Geometry check sheet. Reference: drawing and pictorial views, mm from the part's lowest x, y, z. A direction names the side the tool comes from. Give positions to 0.01 mm unless a question says otherwise; leave off trailing zeros. Write each loop counter-clockwise with the first axis right and the second up, starting at its lowest first coordinate (ties: lowest second). Pieces come first, ordered by that corner, then holes. Notation, with made-up numbers: (7, 0.5) -> (34, 0.5) arc R12 cw to (34, 13.5) -> close; hole circle Ø3 at (-6.75, 10). An arc over 180 degrees is marked (long way). Return JSON: item names as keys, results as strings.
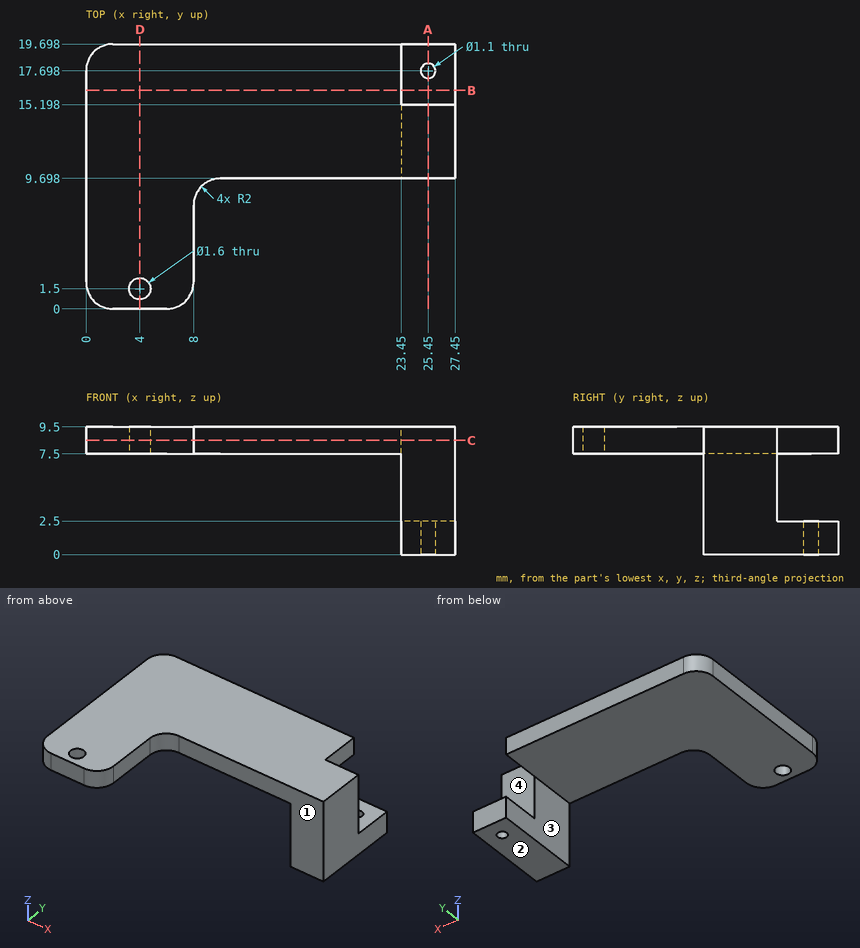
(1) Cross-section at C-C on z = 8.5. Enter the section's corners in (x, y).
Reply:
{"outline": "(0, 2) arc R2 ccw to (2, 0) -> (6, 0) arc R2 ccw to (8, 2) -> (8, 7.7) arc R2 cw to (10, 9.7) -> (27.45, 9.7) -> (27.45, 15.2) -> (23.45, 15.2) -> (23.45, 19.7) -> (2, 19.7) arc R2 ccw to (0, 17.7) -> close; hole circle Ø1.6 at (4, 1.5)"}
(2) Set-up check for the marked faces 1, 2, 3 and 4: record each of +Z, -Z, +X, -X, +Y, -Y from which the full face is reachable in a straight line by a thin tool's end or side.
Reply:
{"face 1": "+Z, -Z, +X, -Y", "face 2": "-Z, +X, -X, +Y, -Y", "face 3": "-Z, -X, +Y, -Y", "face 4": "+Z, +X, +Y"}
(3) Cross-section at D-D on x = 4. Enter the section's corners in (y, z).
Reply:
{"outline": "(0, 7.5) -> (0.7, 7.5) -> (0.7, 9.5) -> (0, 9.5) -> close; (2.3, 7.5) -> (19.7, 7.5) -> (19.7, 9.5) -> (2.3, 9.5) -> close"}
(4) Thickness scan on L1, parallel to Y at x = 4, z = 8.9; L2, parallel to Y at x = 25.45, z = 0.6; L3, parallel to X at y = 12, z = 4.5. Record the ranges inside material, lowest first.
Reply:
{"L1": "0 to 0.7, 2.3 to 19.7", "L2": "9.7 to 17.15, 18.25 to 19.7", "L3": "23.45 to 27.45"}
(5) Cross-section at A-A on x = 25.45. Enter the section's corners in (y, z), then the cut area to 4 significant figures.
Reply:
{"outline": "(9.7, 0) -> (17.15, 0) -> (17.15, 2.5) -> (15.2, 2.5) -> (15.2, 9.5) -> (9.7, 9.5) -> close; (18.25, 0) -> (19.7, 0) -> (19.7, 2.5) -> (18.25, 2.5) -> close", "area": "60.75 mm^2"}
(6) Depth check by flat-ended pin: pin 1 Ø2 at (x, z) = (25.5, 7) entering from +Y; pin 2 Ø1.8 at (x, y) = (4, 1.5) entering from -Z; pin 3 Ø2 at (y, z) = (18, 8.5) entering from +X; pin 4 Ø0.7 at (x, y) = (25.45, 17.698) entering from -Z. Enter the tip coordinate at first touch or a pass-through.
Reply:
{"pin 1": "y = 15.2", "pin 2": "z = 7.5", "pin 3": "x = 23.45", "pin 4": "through"}
(7) Cross-section at B-B on y = 16.25. Enter the section's corners in (x, z), then the cut area to 3 significant figures.
Reply:
{"outline": "(0, 7.5) -> (23.45, 7.5) -> (23.45, 9.5) -> (0, 9.5) -> close; (23.45, 0) -> (27.45, 0) -> (27.45, 2.5) -> (23.45, 2.5) -> close", "area": "56.9 mm^2"}
